from build123d import *

# Parameters (mm, degrees)
F1_DEPTH      = 58
F2_W          = 36
F2_H          = 11
F3_DEPTH      = 63.501
F3_DEPTH_BACK = 63.501
F5_DEPTH      = 38.001


with BuildPart() as f1:
    # F0 (on Front) → F1 (new body)
    with BuildSketch(Plane.XZ):
        with BuildLine():
            Line((-52.5, 9), (-52.5, 0))
            Line((-52.5, 0), (52.5, 0))
            Line((52.5, 0), (52.5, 9))
            Line((52.5, 9), (63.5, 9))
            ThreePointArc((63.5, 9), (55.0060966544, 29.5060966544), (34.5, 38))
            Line((34.5, 38), (-34.5, 38))
            ThreePointArc((-34.5, 38), (-55.0060966544, 29.5060966544), (-63.5, 9))
            Line((-63.5, 9), (-52.5, 9))
        make_face()
    extrude(amount=-F1_DEPTH)

    # F2 (on Right) → F3 (cut, two sides)
    with BuildSketch(Plane.YZ) as f3_sk:
        with Locations((29, 32.5)):
            Rectangle(F2_W, F2_H)
    extrude(amount=-F3_DEPTH, mode=Mode.SUBTRACT)
    extrude(f3_sk.sketch, amount=F3_DEPTH_BACK, mode=Mode.SUBTRACT)

    # F4 (on Top) → F5 (cut, through all)
    with BuildSketch(Plane.XY):
        with BuildLine():
            Line((-33.5, 35.5), (-38.5, 35.5))
            ThreePointArc((-38.5, 35.5), (-45, 29), (-38.5, 22.5))
            Line((-38.5, 22.5), (-33.5, 22.5))
            ThreePointArc((-33.5, 22.5), (-27, 29), (-33.5, 35.5))
        make_face()
        with BuildLine():
            Line((38.5, 35.5), (33.5, 35.5))
            ThreePointArc((33.5, 35.5), (27, 29), (33.5, 22.5))
            Line((33.5, 22.5), (38.5, 22.5))
            ThreePointArc((38.5, 22.5), (45, 29), (38.5, 35.5))
        make_face()
    extrude(amount=F5_DEPTH, mode=Mode.SUBTRACT)


solid = f1.part
Can you work these out from the model? Positions are in its coordinate system, mm. A direction names the side the tool comes from. Give positions to 0.01 mm unless a question says otherwise; leave off trailing zeros. Order: outer loops, then holes, each group sorted by start corner. A loop starts at its lowest first (then second) coordinate and runs counter-clockwise, first axis right, second up. Notation, with made-up numbers: (48.25, -8) - (54.25, -8) arc R30 cw to (54.25, 17) - close; hole circle Ø8 at (44.25, 47). An arc over 180 degrees is marked (long way). Write each question's results on one line, items separated by ' | '.
1) Suppose I cut it at C-C, the plane x = 18. Write out the boundary of the cut face in (y, z), then the cut area to 3 significant figures.
Final values:
outline: (0, 0) - (58, 0) - (58, 38) - (47, 38) - (47, 27) - (11, 27) - (11, 38) - (0, 38) - close | area: 1,810 mm^2
2) Please list where these lines run through material, in increasing order: line 1 along Y through (x, z) = (-16, 28.5); line 2 along Y through (x, z) = (36.5, 17.5); line 3 along X through (y, z) = (24.5, 6.5). Write a range as [from, to].
Final values:
line 1: y = [0, 11], [47, 58] | line 2: y = [0, 22.5], [35.5, 58] | line 3: x = [-52.5, -43.19], [-28.81, 28.81], [43.19, 52.5]
3) On a 3-axis mill with a long thin cutter (end or side, diameter ignored), from which of +Z, -Z, +X, -X, +Y, -Y can I reach the whole of each face in a straight line? I mean faces 1 (the face through (1, 47, 32)), 2 (the face through (-58, 29, 9)), 3 (the face through (52.5, 29, 4)), 4 (the face through (-1, 29, 0)), 5 (the face through (-36, 35.5, 13)). Say none if no direction works.
Final values:
face 1: +Z, +X, -X | face 2: -Z, -X, +Y, -Y | face 3: -Z, +X, +Y, -Y | face 4: -Z, +X, -X, +Y, -Y | face 5: +Z, -Z
4) Suppose I cut it at D-D, the plane z = 31. Write out the boundary of the cut face in (x, y).
Final values:
outline: (-53.39, 0) - (53.39, 0) - (53.39, 11) - (-53.39, 11) - close; (-53.39, 47) - (53.39, 47) - (53.39, 58) - (-53.39, 58) - close
5) Suppose I cut it at B-B, the plane y = 29. Write out the boundary of the cut face in (x, z).
Final values:
outline: (-63.5, 9) - (-52.5, 9) - (-52.5, 0) - (-45, 0) - (-45, 27) - (-57.24, 27) arc R29 ccw to start; (-27, 0) - (27, 0) - (27, 27) - (-27, 27) - close; (45, 0) - (52.5, 0) - (52.5, 9) - (63.5, 9) arc R29 ccw to (57.24, 27) - (45, 27) - close
6) I'm going to push flat-ended pins straight in: pin 1 Ø10 at (y, z) = (43, 26.5) entering from -X; pin 2 Ø3 at (x, y) = (-36, 20.5) entering from +Z; pin 3 Ø5.5 at (x, y) = (58.5, 38) entering from -Z. Where does each tip first touch, or does it pass through?
Final values:
pin 1: stops at x = -60.67 | pin 2: stops at z = 27 | pin 3: stops at z = 9
7) If we mould it in two halves opening along Y, with no side actions, what happens to faces 6 (the face through (36, 35.5, 13)), 7 (the face through (0, 5, 38)), 8 (the face through (-1, 0, 19))? For each: pulls with the +Y half, pulls with the -Y half, needs draft (parallel to the pull), parting line crosses it, or undercut.
Final values:
face 6: undercut | face 7: needs draft | face 8: pulls with the -Y half
8) Suppose I cut it at A-A, the plane z = 5. Write out the boundary of the cut face in (x, y), then the cut area to 3 significant figures.
Final values:
outline: (-52.5, 0) - (52.5, 0) - (52.5, 58) - (-52.5, 58) - close; hole (-38.5, 22.5) - (-33.5, 22.5) arc R6.5 ccw to (-33.5, 35.5) - (-38.5, 35.5) arc R6.5 ccw to start; hole (33.5, 22.5) - (38.5, 22.5) arc R6.5 ccw to (38.5, 35.5) - (33.5, 35.5) arc R6.5 ccw to start | area: 5,690 mm^2
